Verification items for the finished model (mm, model axes). A direction names the side the tool comes from. Round coordinates to 2 decimals unless told otherwise and drop trailing zeros. Write each loop counter-clockwise with the first axis right and the second up, starting at its lowest first coordinate (ties: lowest second). Pieces come first, ordered by that corner, then holes. Notation, with made-up numbers: M 19.5,55 L 29.5,55 A29 cw 29.5,91 Z; hole C 72.25,-21 d1. An arc over 180 degrees is marked long. Write each question's results on one line, items separated by ' | '.
from build123d import *

# Parameters (mm, degrees)
SKETCH1_W                                            = 134
SKETCH1_H                                            = 114
BOSS_EXTRUDE1_DEPTH                                  = 16
SKETCH2_R                                            = 10.5
CUT_EXTRUDE1_DEPTH                                   = 90.409171789
SKETCH3_R                                            = 48
SKETCH3_R_2                                          = 19
CUT_EXTRUDE2_DEPTH                                   = 3
CUT_EXTRUDE3_START                                   = -3
SKETCH5_R                                            = 48
SKETCH5_R_2                                          = 19
CUT_EXTRUDE3_DEPTH                                   = 3
CSK_FOR_M6_HEX_SOCKET_COUNTERSUNK_CAP_SC_D           = 6.6
CSK_FOR_M6_HEX_SOCKET_COUNTERSUNK_CAP_SC_CSINK_D     = 13.44
CSK_FOR_M6_HEX_SOCKET_COUNTERSUNK_CAP_SC_CSINK_ANGLE = 90
SKETCH10_R                                           = 92
CUT_EXTRUDE4_DEPTH                                   = 90.409171789
CUT_EXTRUDE5_DEPTH                                   = 90.409171789
SKETCH13_OUTSIDE_W                                   = 171.332
SKETCH13_OUTSIDE_H                                   = 151.332
CUT_EXTRUDE6_DEPTH                                   = 3
CUT_EXTRUDE7_DEPTH                                   = 90.409171789
CUT_EXTRUDE9_DEPTH                                   = 89.921313531
CUT_EXTRUDE10_DEPTH                                  = 90.409171789
FILLET13_R                                           = 1
FILLET14_R                                           = 1
FILLET16_R                                           = 1
FILLET18_R                                           = 1


with BuildPart() as part:
    # Sketch1 → Boss-Extrude1 (new body)
    with BuildSketch(Plane(origin=(0, 0, 0), x_dir=(1, 0, 0), z_dir=(0, 1, 0))):
        Rectangle(SKETCH1_W, SKETCH1_H)
    extrude(amount=BOSS_EXTRUDE1_DEPTH)

    # Sketch2 → Cut-Extrude1 (cut, through all)
    with BuildSketch(Plane(origin=(0, 16, 0), x_dir=(1, 0, 0), z_dir=(0, 1, 0))):
        with Locations(Location((0, 0, 0), (0, 0, 270))):
            Circle(SKETCH2_R)
    extrude(amount=-CUT_EXTRUDE1_DEPTH, mode=Mode.SUBTRACT)

    # Sketch3 → Cut-Extrude2 (cut)
    with BuildSketch(Plane(origin=(0, 16, 0), x_dir=(1, 0, 0), z_dir=(0, 1, 0))):
        with Locations(Location((0, 0, 0), (0, 0, 270))):
            Circle(SKETCH3_R)
        with Locations(Location((0, 0, 0), (0, 0, 270))):
            Circle(SKETCH3_R_2, mode=Mode.SUBTRACT)
    extrude(amount=-CUT_EXTRUDE2_DEPTH, mode=Mode.SUBTRACT)

    # Sketch5 → Cut-Extrude3 (cut)
    with BuildSketch(Plane.XZ.offset(CUT_EXTRUDE3_START)):
        with Locations(Location((0, 0, 0), (0, 0, 90))):
            Circle(SKETCH5_R)
        with Locations(Location((0, 0, 0), (0, 0, 90))):
            Circle(SKETCH5_R_2, mode=Mode.SUBTRACT)
    extrude(amount=CUT_EXTRUDE3_DEPTH, mode=Mode.SUBTRACT)

    # CSK for M6 Hex Socket Countersunk Cap Screw1 (through all)
    with Locations(Plane(origin=(0, 16, 0), x_dir=(1, 0, 0), z_dir=(0, 1, 0))):
        with Locations((-54, 44), (54, 44), (54, -44), (-54, -44)):
            CounterSinkHole(CSK_FOR_M6_HEX_SOCKET_COUNTERSUNK_CAP_SC_D / 2, CSK_FOR_M6_HEX_SOCKET_COUNTERSUNK_CAP_SC_CSINK_D / 2, counter_sink_angle=CSK_FOR_M6_HEX_SOCKET_COUNTERSUNK_CAP_SC_CSINK_ANGLE)

    # Sketch10 → Cut-Extrude4 (cut, through all)
    with BuildSketch(Plane(origin=(0, 16, 0), x_dir=(1, 0, 0), z_dir=(0, 1, 0))):
        with Locations((149, 0)):
            Circle(SKETCH10_R)
        with Locations((-149, 0)):
            Circle(SKETCH10_R)
    extrude(amount=-CUT_EXTRUDE4_DEPTH, mode=Mode.SUBTRACT)

    # Sketch12 → Cut-Extrude5 (cut, through all)
    with BuildSketch(Plane(origin=(0, 16, 0), x_dir=(1, 0, 0), z_dir=(0, 1, 0))):
        with BuildLine():
            ThreePointArc((-54, -57), (-63.192388155, -53.192388155), (-67, -44))
            Line((-67, -44), (-67, -57))
            Line((-67, -57), (-54, -57))
        make_face()
        with BuildLine():
            ThreePointArc((67, -44), (63.192388155, -53.192388155), (54, -57))
            Line((54, -57), (67, -57))
            Line((67, -57), (67, -44))
        make_face()
        with BuildLine():
            Line((-67, 57), (-67, 44))
            ThreePointArc((-67, 44), (-63.192388155, 53.192388155), (-54, 57))
            Line((-54, 57), (-67, 57))
        make_face()
        with BuildLine():
            Line((67, 57), (54, 57))
            ThreePointArc((54, 57), (63.192388155, 53.192388155), (67, 44))
            Line((67, 44), (67, 57))
        make_face()
    extrude(amount=-CUT_EXTRUDE5_DEPTH, mode=Mode.SUBTRACT)

    # Sketch13 outside → Cut-Extrude6 (cut)
    with BuildSketch(Plane(origin=(0, 16, 0), x_dir=(1, 0, 0), z_dir=(0, 1, 0))):
        Rectangle(SKETCH13_OUTSIDE_W, SKETCH13_OUTSIDE_H)
        with BuildLine():
            ThreePointArc((-51.331145195, 23.980195102), (-56.656176853, -0.117680258), (-51.231084425, -24.193226589))
            ThreePointArc((-51.231084425, -24.193226589), (-51.401784959, -28.792660763), (-55.258927529, -31.303912362))
            ThreePointArc((-55.258927529, -31.303912362), (-63.890720648, -52.059105714), (-41.819855837, -47.797318529))
            ThreePointArc((-41.819855837, -47.797318529), (-38.581301156, -44.526890885), (-34.042183736, -45.288695617))
            ThreePointArc((-34.042183736, -45.288695617), (-0.117680258, -56.656176853), (33.853752972, -45.429721922))
            ThreePointArc((33.853752972, -45.429721922), (38.374825497, -44.679906606), (41.60767448, -47.928138008))
            ThreePointArc((41.60767448, -47.928138008), (64.078054812, -52.211748365), (55.344194725, -31.069681344))
            ThreePointArc((55.344194725, -31.069681344), (51.509943359, -28.559534684), (51.331145195, -23.980195102))
            ThreePointArc((51.331145195, -23.980195102), (56.656299069, 0), (51.331145195, 23.980195102))
            ThreePointArc((51.331145195, 23.980195102), (51.509943359, 28.559534684), (55.344194725, 31.069681344))
            ThreePointArc((55.344194725, 31.069681344), (64.078054812, 52.211748365), (41.60767448, 47.928138008))
            ThreePointArc((41.60767448, 47.928138008), (38.374825497, 44.679906606), (33.853752972, 45.429721922))
            ThreePointArc((33.853752972, 45.429721922), (0, 56.656299069), (-33.853752972, 45.429721922))
            ThreePointArc((-33.853752972, 45.429721922), (-38.374825497, 44.679906606), (-41.60767448, 47.928138008))
            ThreePointArc((-41.60767448, 47.928138008), (-64.078054812, 52.211748365), (-55.344194725, 31.069681344))
            ThreePointArc((-55.344194725, 31.069681344), (-51.509943359, 28.559534684), (-51.331145195, 23.980195102))
        make_face(mode=Mode.SUBTRACT)
    extrude(amount=-CUT_EXTRUDE6_DEPTH, mode=Mode.SUBTRACT)

    # Sketch14 → Cut-Extrude7 (cut, through all)
    with BuildSketch(Plane(origin=(0, 16, 0), x_dir=(1, 0, 0), z_dir=(0, 1, 0))):
        Polygon((67, 44), (66.656381451, 41.030823587), (67, 41.713307229), align=None)
    extrude(amount=-CUT_EXTRUDE7_DEPTH, mode=Mode.SUBTRACT)

    # Sketch15 → Cut-Extrude9 (cut, through all)
    with BuildSketch(Plane(origin=(0, 13, 0), x_dir=(1, 0, 0), z_dir=(0, 1, 0))):
        Polygon((67, -41.713307229), (66.656381451, -41.030823587), (67, -44), align=None)
    extrude(amount=-CUT_EXTRUDE9_DEPTH, mode=Mode.SUBTRACT)

    # Sketch16 → Cut-Extrude10 (cut, through all)
    with BuildSketch(Plane(origin=(0, 16, 0), x_dir=(1, 0, 0), z_dir=(0, 1, 0))):
        Polygon((66.656381451, -41.030823587), (67, -44), (67.112484147, -42.334698628), align=None)
    extrude(amount=-CUT_EXTRUDE10_DEPTH, mode=Mode.SUBTRACT)

    # Fillet13
    fillet13_edges = [part.edges().sort_by_distance(p)[0] for p in [
        (0, 13, -19),
    ]]
    fillet(fillet13_edges, radius=FILLET13_R)

    # Fillet14
    fillet14_edges = [part.edges().sort_by_distance(p)[0] for p in [
        (0, 13, -48),
    ]]
    fillet(fillet14_edges, radius=FILLET14_R)

    # Fillet16
    fillet16_edges = [part.edges().sort_by_distance(p)[0] for p in [
        (0, 3, -19),
    ]]
    fillet(fillet16_edges, radius=FILLET16_R)

    # Fillet18
    fillet18_edges = [part.edges().sort_by_distance(p)[0] for p in [
        (0, 3, -48),
    ]]
    fillet(fillet18_edges, radius=FILLET18_R)


solid = part.part
1) Depth check by flat-ended pin: P1, Ø6, axis at y = 3.5, z = 32.5, coming from the +X side; P2, Ø10.5, axis at x = -54, z = 44, coming from the +Y side; P3, Ø1.5, axis at y = 6, z = -8, coming from the +X side. Enter the tip coordinate at first touch or a pass-through.
Calculated:
P1: stops at x = 64.13 | P2: stops at y = 14.53 | P3: stops at x = 57.42
2) Draft check along X on faces 6 (the flat face through (-6.8, 13, 56.6)), 7 (the cylindrical face through (-51.543, 14.521, -28.617)), 8 (the flat face through (-56.9, 13, 3.2)). Enter one of: pulls with the +X half, pulls with the -X half, needs draft (parallel to the pull), parting line crosses it, or undercut.
Calculated:
face 6: undercut | face 7: pulls with the -X half | face 8: needs draft
3) Access from +Z, -Z, +X, -X, +Y, -Y to the whole of each face (thin tool, end or side, straight path). Record for faces 1 (the cylindrical face through (60.51, 14.521, 32.747)), 2 (the cylindrical face through (0.508, 14.521, -56.654)), 3 (the cylindrical face through (-56.656, 14.521, -0.231)), 4 (the cylindrical face through (11.56, 1.01, -15.08)), 5 (the cylindrical face through (-0.627, 14.521, 56.653)).
Calculated:
face 1: +X, +Y | face 2: -Z, +Y | face 3: -X, +Y | face 4: -Y | face 5: +Z, +Y
4) Material ranges on line 1 (X direction, y = 15.3, z = 0); line 2 (X direction, y = 7.5, z = 44); line 3 (Z direction, x = 54, y = 5), recorded low to high. Write a range as [from, to].
Calculated:
line 1: x = [-56.66, -48], [-19, -10.5], [10.5, 19], [48, 56.66] | line 2: x = [-67, -57.3], [-50.7, 50.7], [57.3, 67] | line 3: z = [-57, -47.3], [-40.7, 40.7], [47.3, 57]
5) Sectioned sample at A-A, the plane y = 6.5. Record the cut outline in (x, z), and give its area (3 significant figures).
Calculated:
outline: M -67,-44 A13 ccw -54,-57 L 54,-57 A13 ccw 67,-44 L 66.66,-41.03 A92 cw 66.66,41.03 L 67,44 A13 ccw 54,57 L -54,57 A13 ccw -67,44 L -67,41.71 A92 cw -67,-41.71 Z; hole C -54,-44 d6.6; hole C -54,44 d6.6; hole C 0,0 d21; hole C 54,-44 d6.6; hole C 54,44 d6.6 | area: 13,500 mm²
